For this review, take the finished solid that the model builds, in its own axes (mm). Face numbers are marked on the shaded views. A direction names the side the tool comes from. Give positions to 0.01 mm unless a question says otherwise; leave off trailing zeros. Loops run counter-clockwise (first coordinate to the right, second up) from the corner with the lowest first, then second, coordinate; pieces in that order, holes last. Notation, with made-up numbers: (50, 55) - (71, 55) arc R27 cw to (71, 81) - close; hole circle Ø4 at (-30.5, 49). An arc over 180 degrees is marked (long way). Answer in a Markdown table with one row per item.
Autodesk Inventor part; units mm, degrees
ref_plane "YZ Plane" through (0, 0, 0) normal (1, 0, 0) x (0, 1, 0)
ref_plane "XZ Plane" through (0, 0, 0) normal (0, 1, 0) x (-1, 0, 0)
ref_plane "XY Plane" through (0, 0, 0) normal (0, 0, 1) x (1, 0, 0)
sketch "Boceto1" plane through (0, 0, 0) normal (0, 1, 0) x (-1, 0, 0)
  line L0 (-6.5, 28) -> (6.5, 28)
  line L1 (6.5, 28) -> (6.5, -28)
  line L2 (6.5, -28) -> (-6.5, -28)
  line L3 (-6.5, -28) -> (-6.5, 28)
  line L4 (-6.5, 28) -> (6.5, -28) construction
  line L5 (6.5, 28) -> (-6.5, -28) construction
  line L6 (5.15, 26.15) -> (-5.15, 26.15)
  line L7 (-5.15, 26.15) -> (-5.15, 13.85)
  line L8 (-5.15, 13.85) -> (5.15, 13.85)
  line L9 (5.15, 13.85) -> (5.15, 26.15)
  line L10 (5.15, 26.15) -> (-5.15, 13.85) construction
  line L11 (-5.15, 26.15) -> (5.15, 13.85) construction
  line L12 (5.15, -13.85) -> (-5.15, -13.85)
  line L13 (-5.15, -13.85) -> (-5.15, -26.15)
  line L14 (-5.15, -26.15) -> (5.15, -26.15)
  line L15 (5.15, -26.15) -> (5.15, -13.85)
  line L16 (5.15, -13.85) -> (-5.15, -26.15) construction
  line L17 (-5.15, -13.85) -> (5.15, -26.15) construction
  point P0 (0, 0)
  point P1 (0, 20)
  point P2 (0, -20)
  point P3 (0, 20)
  point P4 (0, 0)
  point P5 (0, -20)
  point P6 (0, 0)
  dimension "d0" = 12.3
  dimension "d1" = 10.3
  dimension "d2" = 20
  dimension "d3" = 56
  dimension "d4" = 20
  dimension "d5" = 13
extrude "Extrusión1" add sketch "Boceto1" along normal blind 15
sketch "Boceto2" plane through (0, 15, 0) normal (0, 1, 0) x (1, 0, 0)
  line L0 (6.5, 28) -> (-6.5, 28)
  line L1 (-6.5, 28) -> (-6.5, -28)
  line L2 (-6.5, -28) -> (6.5, -28)
  line L3 (6.5, -28) -> (6.5, 28)
  line L4 (-5.15, -26.15) -> (-5.15, -13.85)
  line L5 (-5.15, -13.85) -> (5.15, -13.85)
  line L6 (5.15, -13.85) -> (5.15, -26.15)
  line L7 (5.15, -26.15) -> (-5.15, -26.15)
  line L8 (-5.15, 13.85) -> (-5.15, 26.15)
  line L9 (-5.15, 26.15) -> (5.15, 26.15)
  line L10 (5.15, 26.15) -> (5.15, 13.85)
  line L11 (5.15, 13.85) -> (-5.15, 13.85)
  point P0 (0, 0)
extrude "Extrusión2" add sketch "Boceto2" along normal blind 1 contours L3 L2 L1 L0 | L4 L5 L6 L7 | L8 L9 L10 L11
sketch "Boceto3" plane through (0, 0, 0) normal (0, -1, 0) x (1, 0, 0)
  circle A0 centre (0, 20) radius 2.15
  circle A1 centre (0, -20) radius 2.15
  line L0 (-5.15, 13.85) -> (5.15, 13.85)
  line L1 (5.15, -13.85) -> (-5.15, -13.85)
  line L2 (5.15, 13.85) -> (5.15, 26.15)
  point P0 (0, 0)
  dimension "d10" = 4.3
  dimension "d11" = 6.15
  dimension "d12" = 6.15
  dimension "d13" = 5.15
extrude "Extrusión3" cut sketch "Boceto3" against normal through all
fillet "Empalme1" radius 1.15 8 edges at (5.15, 7.5, -13.85) (5.15, 7.5, 26.15) (5.15, 7.5, 13.85) (5.15, 7.5, -26.15) (-5.15, 7.5, -26.15) (-5.15, 7.5, 13.85) (-5.15, 7.5, -13.85) (-5.15, 7.5, 26.15)
fillet "Empalme2" radius 3 4 edges at (6.5, 8, -28) (6.5, 8, 28) (-6.5, 8, 28) (-6.5, 8, -28)
sketch "Boceto6" plane through (-6.5, 0, -25) normal (-1, 0, 0) x (0, 0, 1)
  line L0 (35.25, -7) -> (14.75, -7)
  line L1 (14.75, -7) -> (14.75, 7)
  line L2 (14.75, 7) -> (35.25, 7)
  line L3 (35.25, 7) -> (35.25, -7)
  line L4 (35.25, -7) -> (14.75, 7) construction
  line L5 (14.75, -7) -> (35.25, 7) construction
  point P0 (25, 0)
  dimension "d30" = 20.5
  dimension "d31" = 7
extrude "Extrusión6" cut sketch "Boceto6" against normal through all
sketch "Boceto7" plane through (0, 16, 0) normal (0, 1, 0) x (1, 0, 0)
  circle A0 centre (0, 0) radius 2.7
  dimension "d35" = 5.4
extrude "Extrusión7" cut sketch "Boceto7" against normal through all
sketch "Boceto8" plane through (0, 0, 0) normal (0, -1, 0) x (1, 0, 0)
  line L0 (4, -13.85) -> (-4, -13.85)
  arc A0 (5.15, -15) -> (4, -13.85) centre (4, -15) ccw
  line L1 (5.15, -25) -> (5.15, -15)
  arc A1 (4, -26.15) -> (5.15, -25) centre (4, -25) ccw
  line L2 (-4, -26.15) -> (4, -26.15)
  arc A2 (-5.15, -25) -> (-4, -26.15) centre (-4, -25) ccw
  line L3 (-5.15, -15) -> (-5.15, -25)
  arc A3 (-4, -13.85) -> (-5.15, -15) centre (-4, -15) ccw
  line L4 (6.5, -10.25) -> (-6.5, -10.25)
  line L5 (-6.5, -25) -> (-6.5, -10.25)
  arc A4 (-6.5, -25) -> (-3.5, -28) centre (-3.5, -25) ccw
  line L6 (3.5, -28) -> (-3.5, -28)
  arc A5 (3.5, -28) -> (6.5, -25) centre (3.5, -25) ccw
  line L7 (6.5, -10.25) -> (6.5, -25)
  line L8 (-6.5, 10.25) -> (6.5, 10.25)
  line L9 (6.5, 25) -> (6.5, 10.25)
  arc A6 (6.5, 25) -> (3.5, 28) centre (3.5, 25) ccw
  line L10 (-3.5, 28) -> (3.5, 28)
  arc A7 (-3.5, 28) -> (-6.5, 25) centre (-3.5, 25) ccw
  line L11 (-6.5, 10.25) -> (-6.5, 25)
  line L12 (4, 26.15) -> (-4, 26.15)
  arc A8 (5.15, 25) -> (4, 26.15) centre (4, 25) ccw
  line L13 (5.15, 15) -> (5.15, 25)
  arc A9 (4, 13.85) -> (5.15, 15) centre (4, 15) ccw
  line L14 (-4, 13.85) -> (4, 13.85)
  arc A10 (-5.15, 15) -> (-4, 13.85) centre (-4, 15) ccw
  line L15 (-5.15, 25) -> (-5.15, 15)
  arc A11 (-4, 26.15) -> (-5.15, 25) centre (-4, 25) ccw
  point P0 (0, 0)
extrude "Extrusión8" cut sketch "Boceto8" against normal blind 4
fillet "Empalme5" radius 1 2 edges at (0, 4, -10.25) (0, 4, 10.25)
sketch "Boceto9" plane through (-6.5, 7, -10.25) normal (0, -1, 0) x (1, 0, 0)
  circle A0 centre (6.5, 10.25) radius 2.7
  line L0 (13, 20.5) -> (13, 0)
  line L1 (0, 20.5) -> (13, 20.5)
  line L2 (0, 0) -> (0, 20.5)
  line L3 (0, 0) -> (13, 0)
  point P0 (6.5, 10.25)
extrude "Extrusión9" cut sketch "Boceto9" against normal blind 0.6
sketch "Boceto4" plane through (0, 16, 0) normal (0, 1, 0) x (1, 0, 0)
  circle A0 centre (0, -5) radius 1.7
  circle A1 centre (0, 5) radius 1.7
  point P0 (0, 0)
  dimension "d19" = 3.4
  dimension "d25" = 5
  dimension "d26" = 5
sketch "Boceto5" plane through (0, 0, 0) normal (0, -1, 0) x (1, 0, 0)
  circle A0 centre (0, 5) radius 1.7
  circle A1 centre (0, 5) radius 2.8
  circle A2 centre (0, -5) radius 1.7
  circle A3 centre (0, -5) radius 2.8
  line L0 (3.2332, 5) -> (1.6166, 2.2)
  line L1 (1.6166, 2.2) -> (-1.6166, 2.2)
  line L2 (-1.6166, 2.2) -> (-3.2332, 5)
  line L3 (-3.2332, 5) -> (-1.6166, 7.8)
  line L4 (-1.6166, 7.8) -> (1.6166, 7.8)
  line L5 (1.6166, 7.8) -> (3.2332, 5)
  line L6 (3.2332, -5) -> (1.6166, -7.8)
  line L7 (1.6166, -7.8) -> (-1.6166, -7.8)
  line L8 (-1.6166, -7.8) -> (-3.2332, -5)
  line L9 (-3.2332, -5) -> (-1.6166, -2.2)
  line L10 (-1.6166, -2.2) -> (1.6166, -2.2)
  line L11 (1.6166, -2.2) -> (3.2332, -5)
  point P0 (0, 0)
  dimension "d27" = 5.6
properties part number "Base"
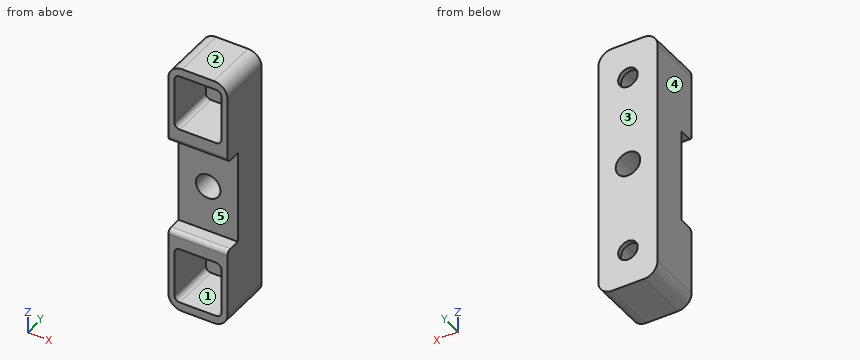
1. Wall thickness on line 1 (Z direction, x = 3, y = 11.75); line 2 (Z direction, x = 0, y = 15.35); line 3 (Z direction, x = 0, y = 14.25): over which ranges is each line inside the solid? List them lowest first. Write a range as [from, to].
Values:
| item | result |
|---|---|
| line 1 | z = [-28, -26.15], [-13.85, 13.85], [26.15, 28] |
| line 2 | z = [-28, -22.15], [-17.85, -2.7], [2.7, 17.85], [22.15, 28] |
| line 3 | z = [-28, -26.15], [-13.85, -2.7], [2.7, 13.85], [26.15, 28] |
2. We need section A-A, the plane x = 0. Count the separate pieces of the cut face and the enclosed holes in it, and give its area (3 significant figures).
Values:
| item | result |
|---|---|
| separate pieces | 4 |
| enclosed holes | 0 |
| area | 273 mm^2 |
3. For the marked faces 1 and 2, list the 3-axis set-ups (+Z, -Z, +X, -X, +Y, -Y) from which the entire face can be reached by the end or side of a thin tool; tool diameter is ignored.
Values:
| item | result |
|---|---|
| face 1 | -Y |
| face 2 | +Z, +X, -X, +Y, -Y |
4. We need section B-B, the plane z = -20. Give the boundary of the cut face in (x, y), and give its area (3 significant figures).
Values:
| item | result |
|---|---|
| outline | (-6.5, 4) - (-5.15, 4) - (-5.15, 15) - (-2.15, 15) - (-2.15, 16) - (-6.5, 16) - close; (2.15, 15) - (5.15, 15) - (5.15, 4) - (6.5, 4) - (6.5, 16) - (2.15, 16) - close |
| area | 38.4 mm^2 |
5. We need section C-C, the plane y = 12. Give the boundary of the cut face in (x, z).
Values:
| item | result |
|---|---|
| outline | (-6.5, -25) arc R3 ccw to (-3.5, -28) - (3.5, -28) arc R3 ccw to (6.5, -25) - (6.5, 25) arc R3 ccw to (3.5, 28) - (-3.5, 28) arc R3 ccw to (-6.5, 25) - close; hole (-5.15, -25) arc R1.15 ccw to (-4, -26.15) - (4, -26.15) arc R1.15 ccw to (5.15, -25) - (5.15, -15) arc R1.15 ccw to (4, -13.85) - (-4, -13.85) arc R1.15 ccw to (-5.15, -15) - close; hole (-5.15, 15) arc R1.15 ccw to (-4, 13.85) - (4, 13.85) arc R1.15 ccw to (5.15, 15) - (5.15, 25) arc R1.15 ccw to (4, 26.15) - (-4, 26.15) arc R1.15 ccw to (-5.15, 25) - close; hole circle Ø5.4 at (0, 0) |
6. Mouldability with a two-part tool opening along Y and no side actions: class the marked faces 3, 4 and 5 as released by +Y, released by -Y, zero draft, split by the parting line, or undercut.
Values:
| item | result |
|---|---|
| face 3 | released by +Y |
| face 4 | zero draft |
| face 5 | released by -Y |
7. Clearance check with flat-ended pins moving along their axes: pin 1 (1 mm diameter, centred on x = -3.5, z = 19.5, fed in from -Y); pin 2 (6.5 mm diameter, centred on x = -2, z = 0, fed in from -Y). State where each tip first meets the part, or that it passes through.
Values:
| item | result |
|---|---|
| pin 1 | stops at y = 15 |
| pin 2 | stops at y = 7.6 |
8. We need section D-D, the plane z = 24.5. Give the boundary of the cut face in (x, y), and give its area (3 significant figures).
Values:
| item | result |
|---|---|
| outline | (-6.5, 4) - (-5.15, 4) - (-5.15, 15) - (5.15, 15) - (5.15, 4) - (6.5, 4) - (6.5, 16) - (-6.5, 16) - close |
| area | 42.7 mm^2 |
